Geometry check sheet. Reference: the model listing, model coordinates, mm. Face numbers are marked on the shaded views. A direction names the side the tool comes from. Give positions to 0.01 mm unless a question says otherwise; leave off trailing zeros. Order: outer loops, then holes, each group sorted by start corner. A loop starts at its lowest first (then second) coordinate and runs counter-clockwise, first axis right, second up. Notation, with made-up numbers: M -29,57.25 L 20,57.25 A9 ccw 20,67.25 Z; hole C 44,-23 d9. An arc over 180 degrees is marked long. One line per question, with ' | ' between items. Start each with the question number.
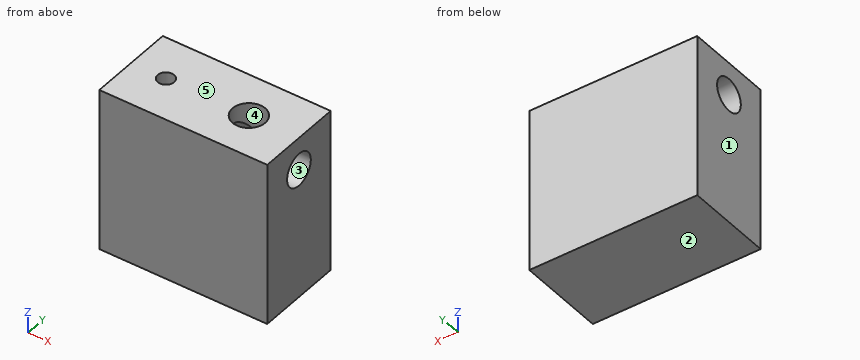
from build123d import *

# Parameters (mm, degrees)
F0_W     = 102.601886
F0_H     = 53.511788
F1_DEPTH = 100
F2_R     = 5
F3_DEPTH = 50
F4_R     = 10
F5_DEPTH = 102.602886
F6_R     = 10
F7_DEPTH = 30


with BuildPart() as f1:
    # F0 (on Top) → F1 (new body)
    with BuildSketch(Plane.XY):
        Rectangle(F0_W, F0_H)
    extrude(amount=F1_DEPTH)

    # F2 (on face) → F3 (cut)
    with BuildSketch(Plane.XY.offset(100)):
        with Locations((-30, 0)):
            Circle(F2_R)
    extrude(amount=-F3_DEPTH, mode=Mode.SUBTRACT)

    # F4 (on face) → F5 (cut, through all)
    with BuildSketch(Plane(origin=(-51.300943, 0, 0), x_dir=(0, -1, 0), z_dir=(-1, 0, 0))):
        with Locations((0, 80)):
            Circle(F4_R)
    extrude(amount=-F5_DEPTH, mode=Mode.SUBTRACT)

    # F6 (on face) → F7 (cut)
    with BuildSketch(Plane.XY.offset(100)):
        with Locations((20.707027, 0)):
            Circle(F6_R)
    extrude(amount=-F7_DEPTH, mode=Mode.SUBTRACT)


solid = f1.part
Item 1: Cross-section at C-C, the plane x = -30. Record the cut outline in (y, z).
Item 2: Material ranges on line 1 along X through (y, z) = (0, 64); line 2 along Y through (x, z) = (43, 80); line 3 along Z through (x, y) = (-24, 0.5), recorded low to high.
Item 3: Cross-section at B-B, the plane z = 86. Record the cut outline in (x, y).
Item 4: Set-up check for the marked faces 4 and 5: record each of +Z, -Z, +X, -X, +Y, -Y from which the full face is reachable in a straight line by a thin tool's end or side.
Item 5: Mould release check, pull along Z, two halves, no side actions. Record for the marked faces 1, 2 and 3: released by +Z, released by -Z, zero draft, split by the parting line, or undercut.
Item 6: Cross-section at A-A, the plane x = 42. Record the cut outline in (y, z).
Item 7: Depth check by flat-ended pin: pin 1 (6 mm diameter, centred on x = 19, y = 2.5, fed in from +Z); pin 2 (3 mm diameter, centred on x = -32, y = 2, fed in from +Z). Enter the tip coordinate at first touch or a pass-through.
Item 8: Cross-section at D-D, the plane x = 18.5. Record the cut outline in (y, z).
Outcome:
1) outline: M -26.76,0 L 26.76,0 L 26.76,100 L 5,100 L 5,88.66 A10 cw 5,71.34 L 5,50 L -5,50 L -5,71.34 A10 cw -5,88.66 L -5,100 L -26.76,100 Z
2) line 1: x = -51.3 to -35, -25 to 51.3 | line 2: y = -26.76 to -10, 10 to 26.76 | line 3: z = 0 to 70.01, 89.99 to 100
3) outline: M -51.3,-26.76 L 51.3,-26.76 L 51.3,-8 L 26.71,-8 A10 cw 14.71,-8 L -51.3,-8 Z; M -51.3,8 L 14.71,8 A10 cw 26.71,8 L 51.3,8 L 51.3,26.76 L -51.3,26.76 Z
4) face 4: +Z | face 5: +Z, +X, -X, +Y, -Y
5) face 1: zero draft | face 2: released by -Z | face 3: undercut
6) outline: M -26.76,0 L 26.76,0 L 26.76,100 L -26.76,100 Z; hole C 0,80 d20
7) pin 1: stops at z = 70 | pin 2: stops at z = 50
8) outline: M -26.76,0 L 26.76,0 L 26.76,100 L 9.75,100 L 9.75,82.21 A10 cw 9.75,77.79 L 9.75,70 L -9.75,70 L -9.75,77.79 A10 cw -9.75,82.21 L -9.75,100 L -26.76,100 Z
